Check sheet for the modelled part. Datum: model origin and axes. Units: mm. A direction names the side the tool comes from. Round coordinates to 2 decimals unless told otherwise and drop trailing zeros. Order: outer loops, then holes, each group sorted by start corner. A loop starts at its lowest first (then second) coordinate and runs counter-clockwise, first axis right, second up.
Q1. Set-up check for faces 4 (the flat face through (8.34, -1.62, -30.2)), 5 (the flat face through (-2.871, -17.803, -32.843)), 6 (the flat face through (-2.87, -0.2, -32.85)), 7 (the flat face through (0, -9, -15)), 8 (the flat face through (10, -9, -32)): record each of +Z, -Z, +X, -X, +Y, -Y from which the full face is reachable in a straight line by a thin tool's end or side.
Q2. Cross-section at D-D on z = -4. Record the cut outline in (x, y), then the cut area to 3 significant figures.
Q3. Cross-section at B-B on y = -9. Give the number of separate pieces and of enclosed holes in the cut face, then the cut area to 3 significant figures.
Q4. Scan lines: probe 1 along X at (y, z) = (-9, 1); probe 2 along Y at (x, z) = (20, 2); probe 3 along X at (y, z) = (-9, 3.15). Record each from-to range of solid material in increasing order.
Q5. Depth check by flat-ended pin: P1, Ø4.5, axis at x = 75, y = -9, coming from the +Z side; P2, Ø5, axis at x = 16.5, y = -11, coming from the -Z side; P3, Ø2.5, axis at y = -8, z = -31.5, coming from the +X side; P4, Ø5, axis at y = -12, z = -16, coming from the +X side. Enter the tip coordinate at first touch or a pass-through.
Q6. Cross-section at A-A on x = 75. Record the cut outline in (y, z), then the cut area to 3 significant figures.
Q7. Mould release check, pull along X, two halves, no side actions. Record for faces 1 (the flat face through (-2.843, -17.803, 2.871)), 2 (the flat face through (9, -2, -32)), 3 (the cylindrical face through (21.508, -7.844, 2.225)): +X half, -X half, draft (parallel to the pull), parting line (faces both ways), or undercut.
Q8. Cross-section at C-C on x = 54.5. Record the cut outline in (y, z).
from build123d import *

# Parameters (mm, degrees)
PAD003_DEPTH       = 18
SKETCH010_R        = 1.9
SKETCH010_R_2      = 1.65
POCKET007_DEPTH    = 5
SKETCH011_R        = 3.5
POCKET008_DEPTH    = 2
CHAMFER012008_SIZE = 3
CHAMFER012009_SIZE = 2
CHAMFER012010_SIZE = 0.4
CHAMFER012011_SIZE = 0.4


with BuildPart() as part:
    # Sketch009 → Pad003 (new body)
    with BuildSketch(Plane.XZ):
        Polygon((0, 0), (79.2, 0), (79.2, 4), (-4, 4), (-4, -34), (10, -34), (10, -30), (0, -30), align=None)
    extrude(amount=PAD003_DEPTH)

    # Sketch010 (on Face3 of Pad003) → Pocket007 (cut)
    with BuildSketch(Plane(origin=(0, 0, 4), x_dir=(-1, 0, 0), z_dir=(0, 0, 1))):
        with Locations((-75, 9)):
            Circle(SKETCH010_R)
        with Locations((-65, 9)):
            Circle(SKETCH010_R_2)
        with Locations((-20, 9)):
            Circle(SKETCH010_R)
    extrude(amount=-POCKET007_DEPTH, mode=Mode.SUBTRACT)

    # Sketch011 (on Face10 of Pocket007) → Pocket008 (cut)
    with BuildSketch(Plane(origin=(0, 0, 4), x_dir=(-1, 0, 0), z_dir=(0, 0, 1))):
        with Locations((-65, 9)):
            Circle(SKETCH011_R)
    extrude(amount=-POCKET008_DEPTH, mode=Mode.SUBTRACT)

    # Chamfer012008
    chamfer012008_edges = [part.edges().sort_by_distance(p)[0] for p in [
        (10, -18, -32),
        (10, 0, -32),
        (79.2, -18, 2),
        (79.2, 0, 2),
    ]]
    chamfer(chamfer012008_edges, length=CHAMFER012008_SIZE)

    # Chamfer012009
    chamfer012009_edges = [part.edges().sort_by_distance(p)[0] for p in [
        (-4, -9, -34),
        (-4, -9, 4),
    ]]
    chamfer(chamfer012009_edges, length=CHAMFER012009_SIZE)

    # Chamfer012010
    chamfer012010_edges = [part.edges().sort_by_distance(p)[0] for p in [
        (8.5, -16.5, -34),
        (7, -18, -32),
        (10, -15, -32),
        (8.5, -16.5, -30),
        (10, -9, -34),
        (10, -3, -32),
        (10, -9, -30),
        (37.1, -18, 4),
        (-3, -18, 3),
        (76.2, -18, 2),
        (-4, -18, -15),
        (38.1, -18, 0),
        (-3, -18, -33),
        (0, -18, -15),
        (2.5, -18, -34),
        (3.5, -18, -30),
        (77.7, -16.5, 0),
        (79.2, -15, 2),
        (77.7, -16.5, 4),
        (79.2, -9, 0),
        (79.2, -3, 2),
        (79.2, -9, 4),
        (77.7, -1.5, 0),
        (76.2, 0, 2),
        (77.7, -1.5, 4),
        (37.1, 0, 4),
        (-3, 0, 3),
        (-4, 0, -15),
        (38.1, 0, 0),
        (-3, 0, -33),
        (0, 0, -15),
        (2.5, 0, -34),
        (3.5, 0, -30),
        (7, 0, -32),
        (8.5, -1.5, -34),
        (8.5, -1.5, -30),
    ]]
    chamfer(chamfer012010_edges, length=CHAMFER012010_SIZE)

    # Chamfer012011
    chamfer012011_edges = [part.edges().sort_by_distance(p)[0] for p in [
        (21.9, -9, 0),
        (76.9, -9, 0),
    ]]
    chamfer(chamfer012011_edges, length=CHAMFER012011_SIZE)


solid = part.part
Results found:
1. face 4: +X, +Y
1. face 5: -Z, -X, -Y
1. face 6: -Z, -X, +Y
1. face 7: +X, +Y, -Y
1. face 8: -Z, +X, +Y, -Y
2. outline: (-4, -17.6) - (-3.6, -18) - (-0.4, -18) - (0, -17.6) - (0, -0.4) - (-0.4, 0) - (-3.6, 0) - (-4, -0.4) - close
2. area: 71.7 mm2
3. separate pieces: 4
3. enclosed holes: 0
3. area: 453 mm2
4. probe 1: x = -4 to 18.1, 21.9 to 63.35, 66.65 to 73.1, 76.9 to 79.2
4. probe 2: y = -18 to -10.9, -7.1 to 0
4. probe 3: x = -2.85 to 18.1, 21.9 to 61.5, 68.5 to 73.1, 76.9 to 79.2
5. P1: stops at z = 4
5. P2: stops at z = 0
5. P3: stops at x = 10
5. P4: stops at x = 0
6. outline: (-18, 0.4) - (-17.6, 0) - (-11.3, 0) - (-10.9, 0.4) - (-10.9, 4) - (-17.6, 4) - (-18, 3.6) - close; (-7.1, 0.4) - (-6.7, 0) - (-0.4, 0) - (0, 0.4) - (0, 3.6) - (-0.4, 4) - (-7.1, 4) - close
6. area: 56.3 mm2
7. face 1: -X half
7. face 2: +X half
7. face 3: undercut
8. outline: (-18, 0.4) - (-17.6, 0) - (-0.4, 0) - (0, 0.4) - (0, 3.6) - (-0.4, 4) - (-17.6, 4) - (-18, 3.6) - close
